```python
from build123d import *

# Parameters (mm, degrees)
SKETCH1_R           = 30
SKETCH1_R_2         = 2
BOSS_EXTRUDE1_DEPTH = 7
SKETCH2_R           = 12.5
BOSS_EXTRUDE2_DEPTH = 7
SKETCH3_R           = 12.5
BOSS_EXTRUDE3_DEPTH = 7


with BuildPart() as part:
    # Sketch1 → Boss-Extrude1 (new body)
    with BuildSketch(Plane(origin=(0, 0, 0), x_dir=(1, 0, 0), z_dir=(0, 1, 0))):
        with Locations(Location((0, 0, 0), (0, 0, 270))):
            Circle(SKETCH1_R)
        with Locations(Location((0, 25, 0), (0, 0, 270))):
            Circle(SKETCH1_R_2, mode=Mode.SUBTRACT)
        with Locations(Location((21.650635095, 12.5, 0), (0, 0, 270))):
            Circle(SKETCH1_R_2, mode=Mode.SUBTRACT)
        with Locations(Location((21.650635095, -12.5, 0), (0, 0, 270))):
            Circle(SKETCH1_R_2, mode=Mode.SUBTRACT)
        with Locations(Location((0, -25, 0), (0, 0, 270))):
            Circle(SKETCH1_R_2, mode=Mode.SUBTRACT)
        with Locations(Location((-21.650635095, -12.5, 0), (0, 0, 270))):
            Circle(SKETCH1_R_2, mode=Mode.SUBTRACT)
        with Locations(Location((-21.650635095, 12.5, 0), (0, 0, 270))):
            Circle(SKETCH1_R_2, mode=Mode.SUBTRACT)
    extrude(amount=BOSS_EXTRUDE1_DEPTH)

    # Sketch2 → Boss-Extrude2 (add)
    with BuildSketch(Plane(origin=(0, 7, 0), x_dir=(1, 0, 0), z_dir=(0, 1, 0))):
        with Locations(Location((-0.5, 0, 0), (0, 0, 270))):
            Circle(SKETCH2_R)
    extrude(amount=BOSS_EXTRUDE2_DEPTH)

    # Sketch3 → Boss-Extrude3 (add)
    with BuildSketch(Plane(origin=(0, 14, 0), x_dir=(1, 0, 0), z_dir=(0, 1, 0))):
        with Locations(Location((0.5, 0, 0), (0, 0, 92.292442776))):
            Circle(SKETCH3_R)
    extrude(amount=BOSS_EXTRUDE3_DEPTH)


solid = part.part
```
Geometry: final body of the model. Coordinates: model frame, mm. A direction names the side the tool comes from. Round coordinates to 2 decimals unless told otherwise and drop trailing zeros. Loops run counter-clockwise (first coordinate to the right, second up) from the corner with the lowest first, then second, coordinate; pieces in that order, holes last. Notation, with made-up numbers: (-31.5, 67) -> (25.5, 67) arc R22 ccw to (25.5, 87) -> close; hole circle Ø11 at (72, 37.25). An arc over 180 degrees is marked (long way). Use one line per item in the form item = value. Start each with the question number.
1) Section D-D on x = 22.5. Output: boundary loops of the cut face in (y, z).
2) Section A-A on z = -25. Output: boundary loops of the cut face in (x, y).
3) Section B-B on z = 0. Output: boundary loops of the cut face in (x, y), then the cut area to 3 significant figures.
4) Access query for faces 1 (the cylindrical face through (12.8, 17.45, 2.22)), 2 (the flat face through (-12.2, 14, -0.1)), 3 (the flat face through (0, 0, 0)), 4 (the cylindrical face through (-23.603, 3.451, 12.066)), 5 (the cylindrical face through (3, 10, 12)). Directions: +Z, -Z, +X, -X, +Y, -Y. A direction counts if a zero-diameter tool reaches every point of the face in a straight line with its end or side. Return the directions, or none.
5) Line query: L1, parallel to X at y = 4, z = -12.5; L2, parallel to Y at x = 21, z = 16; L3, parallel to X at y = 5, z = -26.5. Output: solid intervals per line, ascending.
6) Draft query along Y for faces 6 (the cylindrical face through (-1.2, 3.5, 23.4)), 7 (the flat face through (12.2, 14, -0.4)), 8 (the flat face through (0, 21, 0)). Return one class per face: released by +Y, released by -Y, zero draft, split by the parting line, or undercut.
7) First-contact query: P1, Ø6.5, axis at x = -21.65, z = -12.5, coming from the +Y side; P2, Ø2, axis at y = 9.5, z = -1, coming from the +X side; P3, Ø2, axis at x = -15.5, y = 2.5, coming from the +Z side. Flat tips, straight axial feed; report the tip coordinate or a pass-through.
8) Section C-C on y = 3.5. Output: boundary loops of the cut face in (x, z).
Response:
q1.outline = (0, -19.84) -> (7, -19.84) -> (7, -14.31) -> (0, -14.31) -> close; (0, -10.69) -> (7, -10.69) -> (7, 10.69) -> (0, 10.69) -> close; (0, 14.31) -> (7, 14.31) -> (7, 19.84) -> (0, 19.84) -> close
q2.outline = (-16.58, 0) -> (-2, 0) -> (-2, 7) -> (-16.58, 7) -> close; (2, 0) -> (16.58, 0) -> (16.58, 7) -> (2, 7) -> close
q3.outline = (-30, 0) -> (30, 0) -> (30, 7) -> (12, 7) -> (12, 14) -> (13, 14) -> (13, 21) -> (-12, 21) -> (-12, 14) -> (-13, 14) -> (-13, 7) -> (-30, 7) -> close
q3.area = 770 mm^2
q4.face_1 = +Y
q4.face_2 = -X, +Y
q4.face_3 = +Z, -Z, +X, -X, -Y
q4.face_4 = +Y, -Y
q4.face_5 = none
q5.L1 = -27.27 to -23.65, -19.65 to 19.65, 23.65 to 27.27
q5.L2 = 0 to 7
q5.L3 = -14.06 to -1.32, 1.32 to 14.06
q6.face_6 = zero draft
q6.face_7 = undercut
q6.face_8 = released by +Y
q7.P1 = 7
q7.P2 = 12
q7.P3 = 26.26
q8.outline = circle Ø60 at (0, 0); hole circle Ø4 at (-21.65, -12.5); hole circle Ø4 at (-21.65, 12.5); hole circle Ø4 at (0, -25); hole circle Ø4 at (0, 25); hole circle Ø4 at (21.65, -12.5); hole circle Ø4 at (21.65, 12.5)
